Could you check a few things on this drawing? It's one solid part, dimensions in mm from its lowest x, y, z. Give positions to 0.01 mm unless a question says otherwise; leave off trailing zeros. Loops run counter-clockwise (first coordinate to the right, second up) from the corner with the lowest first, then second, coordinate; pieces in that order, holes last. Notation, with made-up numbers: M 62.5,-3 L 69.5,-3 A17 ccw 69.5,8 Z; hole C -16.5,62.25 d9. An arc over 180 degrees is marked long. Answer as CSV lines item,"result". Start each with the question number.
Item 1: I want a section at D-D on z = 43. List the corners of the cut face in (x, y) for me, plus the area to 3 significant figures.
Item 2: If I drill on line 1 along Z through (x, y) = (5, 3.5); line 2 along X through (y, z) = (1.85, 56.25); line 3 along X through (y, z) = (1.6, 4), over which ranges is the centre line in solid material (lowest first)? Write a range as from..to.
Item 3: I want a section at B-B on y = 1.6. List the corners of the cut face in (x, z) for me.
Item 4: I want a section at C-C on x = 10.25. List the corners of the cut face in (y, z) for me, plus the area to 3 significant figures.
Item 5: I want a section at A-A on x = 4. List the corners of the cut face in (y, z) for me, plus the area to 3 significant figures.
Item 6: Will these pins go through, and if not, where does the flat tip stop? P1, Ø2, axis at y = 1.5, z = 66.5, coming from the +X side; P2, Ø1, axis at x = 14.5, y = 3, coming from the +Z side.
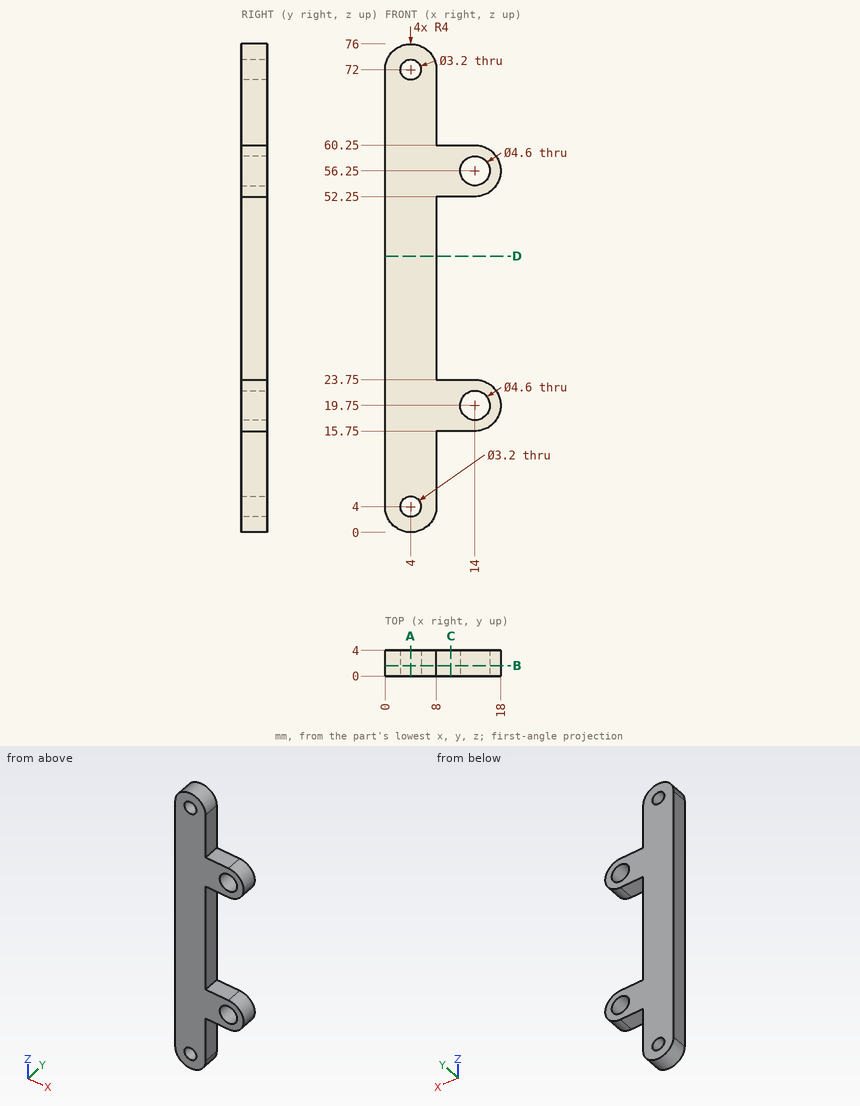
Result:
1,outline,"M 0,0 L 8,0 L 8,4 L 0,4 Z"
1,area,"32.0 mm^2"
2,line 1,"0.13..2.75, 5.25..70.75, 73.25..75.87"
2,line 2,"0..11.7, 16.3..18"
2,line 3,"0..2.4, 5.6..8"
3,outline,"M 0,4 A4 ccw 8,4 L 8,15.75 L 14,15.75 A4 ccw 14,23.75 L 8,23.75 L 8,52.25 L 14,52.25 A4 ccw 14,60.25 L 8,60.25 L 8,72 A4 ccw 0,72 Z; hole C 4,4 d3.2; hole C 4,72 d3.2; hole C 14,19.75 d4.6; hole C 14,56.25 d4.6"
4,outline,"M 0,15.75 L 4,15.75 L 4,23.75 L 0,23.75 Z; M 0,52.25 L 4,52.25 L 4,60.25 L 0,60.25 Z"
4,area,"64.0 mm^2"
5,outline,"M 0,0 L 4,0 L 4,2.4 L 0,2.4 Z; M 0,5.6 L 4,5.6 L 4,70.4 L 0,70.4 Z; M 0,73.6 L 4,73.6 L 4,76 L 0,76 Z"
5,area,"278 mm^2"
6,P1,"x = 8"
6,P2,"z = 60.25"
